```python
from build123d import *

# Parameters (mm, degrees)
F0_W     = 84
F0_H     = 9
F0_R     = 1.25
F0_W_2   = 72
F0_H_2   = 3
F1_DEPTH = 2


with BuildPart() as f1:
    # F0 (on Front) → F1 (new body)
    with BuildSketch(Plane.XZ):
        Rectangle(F0_W, F0_H)
        with Locations((-37.5, 0)):
            Circle(F0_R, mode=Mode.SUBTRACT)
        with Locations((3, 0)):
            Rectangle(F0_W_2, F0_H_2, mode=Mode.SUBTRACT)
        Polygon((45, 4.5), (42, 4.5), (42, -4.5), (42, -13.5), (45, -13.5), align=None)
        Polygon((-42, -4.5), (-42, 4.5), (-45, 4.5), (-45, -13.5), (-42, -13.5), align=None)
        with Locations((0, -9)):
            Rectangle(F0_W, F0_H)
        with Locations((-31.5, -9)):
            Circle(F0_R, mode=Mode.SUBTRACT)
        with Locations((0, -9)):
            Circle(F0_R, mode=Mode.SUBTRACT)
        with Locations((31.5, -9)):
            Circle(F0_R, mode=Mode.SUBTRACT)
    extrude(amount=F1_DEPTH)


solid = f1.part
```
Model file for the job. Use its own axes, mm. A direction names the side the tool comes from. Round coordinates to 2 decimals unless told otherwise and drop trailing zeros. Write each loop counter-clockwise with the first axis right and the second up, starting at its lowest first coordinate (ties: lowest second). Pieces come first, ordered by that corner, then holes. Notation, with made-up numbers: (-19.75, 60) -> (-9.75, 60) arc R30 cw to (-9.75, 91) -> close; hole circle Ø1 at (28.5, -12.5). An arc over 180 degrees is marked (long way). Answer as CSV lines item,"result".
1. Slice it at D-D, the plane z = -9. List the corners of the cut face in (x, y), plus the area to 3 significant figures.
Resolved:
outline,"(-45, -2) -> (-32.75, -2) -> (-32.75, 0) -> (-45, 0) -> close; (-30.25, -2) -> (-1.25, -2) -> (-1.25, 0) -> (-30.25, 0) -> close; (1.25, -2) -> (30.25, -2) -> (30.25, 0) -> (1.25, 0) -> close; (32.75, -2) -> (45, -2) -> (45, 0) -> (32.75, 0) -> close"
area,"165 mm²"
2. Drill centre lines: line 1 (Z direction, x = 31.5, y = -1.2); line 2 (Z direction, x = 24, y = -1.05); line 3 (Z direction, x = 32, y = -1.5). Where is each one in solid material? Low to high.
Resolved:
line 1,"-13.5 to -10.25, -7.75 to -1.5, 1.5 to 4.5"
line 2,"-13.5 to -1.5, 1.5 to 4.5"
line 3,"-13.5 to -10.15, -7.85 to -1.5, 1.5 to 4.5"
3. Pin check, flat tip, straight feed: pin 1 Ø2 at (x, z) = (-37.5, 0) entering from -Y. Stop position of the tip, or through.
Resolved:
pin 1,"through"
4. Slice it at C-C, the plane y = -0.7. List the corners of the cut face in (x, z), plus the area to 3 significant figures.
Resolved:
outline,"(-45, -13.5) -> (45, -13.5) -> (45, 4.5) -> (-45, 4.5) -> close; hole circle Ø2.5 at (-37.5, 0); hole (-33, -1.5) -> (39, -1.5) -> (39, 1.5) -> (-33, 1.5) -> close; hole circle Ø2.5 at (-31.5, -9); hole circle Ø2.5 at (0, -9); hole circle Ø2.5 at (31.5, -9)"
area,"1,380 mm²"
5. Mould opens along X. For faces 3 (the face through (32.69, -0.99, -8.62)), 4 (the face through (-45, -1, -4)), 5 (the face through (1, -1, 4.5)) say: +X half, -X half, draft (parallel to the pull), parting line (faces both ways), or undercut.
Resolved:
face 3,"undercut"
face 4,"-X half"
face 5,"draft"
6. Tool access for faces 1 (the face through (2, -1, -1.5)), 2 (the face through (-1, -2, -4)): list every direction of +Z, -Z, +X, -X, +Y, -Y with a clear straight run to the whole face (end or side of a thin tool).
Resolved:
face 1,"+Y, -Y"
face 2,"+Z, -Z, +X, -X, -Y"
7. Slice it at B-B, the plane x = -31.5. List the corners of the cut face in (y, z), plus the area to 3 significant figures.
Resolved:
outline,"(-2, -13.5) -> (0, -13.5) -> (0, -10.25) -> (-2, -10.25) -> close; (-2, -7.75) -> (0, -7.75) -> (0, -1.5) -> (-2, -1.5) -> close; (-2, 1.5) -> (0, 1.5) -> (0, 4.5) -> (-2, 4.5) -> close"
area,"25.0 mm²"
8. Slice it at A-A, the plane z = 0. List the corners of the cut face in (x, y), plus the area to 3 significant figures.
Resolved:
outline,"(-45, -2) -> (-38.75, -2) -> (-38.75, 0) -> (-45, 0) -> close; (-36.25, -2) -> (-33, -2) -> (-33, 0) -> (-36.25, 0) -> close; (39, -2) -> (45, -2) -> (45, 0) -> (39, 0) -> close"
area,"31.0 mm²"
